from build123d import *

# Parameters (mm, degrees)
BOSS_EXTRUDE1_DEPTH = 101.6
SKETCH3_R           = 3.175
CUT_EXTRUDE1_DEPTH  = 113.208291249


with BuildPart() as part:
    # Sketch1 → Boss-Extrude1 (new body)
    with BuildSketch(Plane(origin=(0, 0, 0), x_dir=(1, 0, 0), z_dir=(0, 1, 0))):
        Polygon((0, 0), (0, 28.575), (3.175, 28.575), (3.175, 3.175), (34.925, 3.175), (34.925, 28.575), (38.1, 28.575), (38.1, 0), align=None)
    extrude(amount=BOSS_EXTRUDE1_DEPTH)

    # Sketch3 → Cut-Extrude1 (cut, through all)
    with BuildSketch(Plane.ZY):
        with Locations((-16.66875, 12.7)):
            Circle(SKETCH3_R)
        with Locations((-16.66875, 38.1)):
            Circle(SKETCH3_R)
        with Locations((-16.66875, 63.5)):
            Circle(SKETCH3_R)
        with Locations((-16.66875, 88.9)):
            Circle(SKETCH3_R)
    extrude(amount=-CUT_EXTRUDE1_DEPTH, mode=Mode.SUBTRACT)


solid = part.part
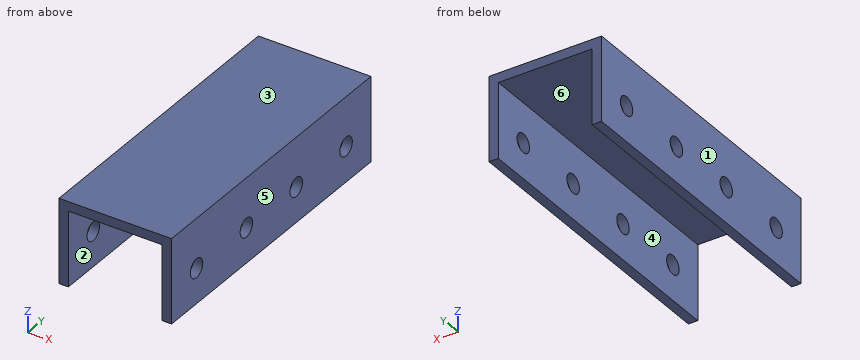
Read the model definition and answer for the solid it produces. Units are mm, in the model's axes. Face numbers are marked on the shaded views. A direction names the side the tool comes from. Round coordinates to 2 decimals unless told otherwise and drop trailing zeros. Write each loop counter-clockwise with the first axis right and the second up, starting at its lowest first coordinate (ties: lowest second). Pieces come first, ordered by that corner, then holes.
1. The part is cut by section C-C, the plane y = 51.5. Determine the outline of the cut face in (x, z) (3 decimals), then the cut area to 3 significant figures.
2. Given pin 1 Ø5.5 at (y, z) = (38.1, -16.67) entering from -X, flat-ended and moving along its own axis, determine where the tip first touches the part or whether it passes through.
3. Which of the six approach directions +Z, -Z, +X, -X, +Y, -Y give full straight-line access (tool end or side, diameter ignored) to the marked faces 5 and 6?
4. The part is cut by section D-D, the plane x = 15.5. Determine the outline of the cut face in (y, z) (3 decimals), then the cut area to 3 significant figures.
5. The part is cut by section B-B, the plane y = 88.9. Determine the outline of the cut face in (x, z) (3 decimals), then the cut area to 3 significant figures.
6. The part is cut by section A-A, the plane z = -22. Determine the outline of the cut face in (x, y) (3 decimals), then the cut area to 3 significant figures.
7. Straight lines are drawn through the part: L1, parallel to X at y = 91, z = -25.5 (3 decimals); L2, parallel to Z at x = 35, y = 12 (3 decimals); L3, parallel to Z at x = 23, y = 31.5 (3 decimals). For each, find the intervals that lie inside material, in ascending order.
8. Determine the mould class of the marked faces 1, 2, 3 and 4 for opening direction X: pulls with the +X half, pulls with the -X half, needs draft (parallel to the pull), parting line crosses it, or undercut.
Values:
1. outline: (0, -28.575) - (3.175, -28.575) - (3.175, -3.175) - (34.925, -3.175) - (34.925, -28.575) - (38.1, -28.575) - (38.1, 0) - (0, 0) - close
1. area: 282 mm2
2. pin 1: passes through
3. face 5: +Z, -Z, +X, +Y, -Y
3. face 6: -Z, +Y, -Y
4. outline: (0, -3.175) - (101.6, -3.175) - (101.6, 0) - (0, 0) - close
4. area: 323 mm2
5. outline: (0, -28.575) - (3.175, -28.575) - (3.175, -19.844) - (0, -19.844) - close; (0, -13.494) - (3.175, -13.494) - (3.175, -3.175) - (34.925, -3.175) - (34.925, -13.494) - (38.1, -13.494) - (38.1, 0) - (0, 0) - close; (34.925, -28.575) - (38.1, -28.575) - (38.1, -19.844) - (34.925, -19.844) - close
5. area: 242 mm2
6. outline: (0, 0) - (3.175, 0) - (3.175, 101.6) - (0, 101.6) - close; (34.925, 0) - (38.1, 0) - (38.1, 101.6) - (34.925, 101.6) - close
6. area: 645 mm2
7. L1: x = 0 to 3.175, 34.925 to 38.1
7. L2: z = -28.575 to -19.766, -13.572 to 0
7. L3: z = -3.175 to 0
8. face 1: pulls with the -X half
8. face 2: undercut
8. face 3: needs draft
8. face 4: undercut
